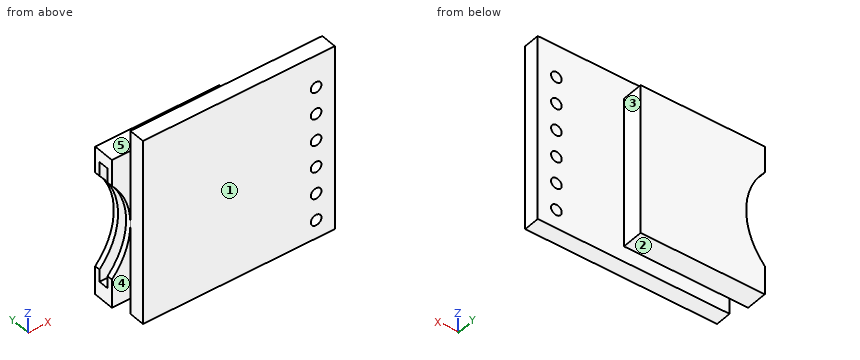
from build123d import *

# Parameters (mm, degrees)
SKETCH1_W           = 18
SKETCH1_H           = 17.5
BOSS_EXTRUDE1_DEPTH = 1.5
BOSS_EXTRUDE2_DEPTH = 2
SKETCH3_R           = 0.5
CUT_EXTRUDE1_DEPTH  = 2.5
SKETCH4_W           = 11.451958773
SKETCH4_H           = 0.968573627
CUT_EXTRUDE2_DEPTH  = 9.649638


with BuildPart() as part:
    # Sketch1 → Boss-Extrude1 (new body)
    with BuildSketch(Plane(origin=(0, 0, 0), x_dir=(1, 0, 0), z_dir=(0, 1, 0))):
        with Locations((9, 8.75)):
            Rectangle(SKETCH1_W, SKETCH1_H)
    extrude(amount=BOSS_EXTRUDE1_DEPTH)

    # Sketch2 → Boss-Extrude2 (add)
    with BuildSketch(Plane(origin=(0, 1.5, 0), x_dir=(1, 0, 0), z_dir=(0, 1, 0))):
        with BuildLine():
            Line((-1.742375604, 4.397064227), (-1.742375604, 1.912224032))
            Line((-1.742375604, 1.912224032), (9.907262148, 1.912224032))
            Line((9.907262148, 1.912224032), (9.907262148, 16.039286602))
            Line((9.907262148, 16.039286602), (-1.742375604, 16.039286602))
            Line((-1.742375604, 16.039286602), (-1.742375604, 13.34923012))
            ThreePointArc((-1.742375604, 13.34923012), (0, 8.873147173), (-1.742375604, 4.397064227))
        make_face()
    extrude(amount=BOSS_EXTRUDE2_DEPTH)

    # Sketch3 → Cut-Extrude1 (cut, through all)
    with BuildSketch(Plane(origin=(0, 1.5, 0), x_dir=(1, 0, 0), z_dir=(0, 1, 0))):
        with Locations((16.25, 15.75)):
            Circle(SKETCH3_R)
        with Locations((16.25, 13.21)):
            Circle(SKETCH3_R)
        with Locations((16.25, 10.67)):
            Circle(SKETCH3_R)
        with Locations((16.25, 8.13)):
            Circle(SKETCH3_R)
        with Locations((16.25, 5.59)):
            Circle(SKETCH3_R)
        with Locations((16.25, 3.05)):
            Circle(SKETCH3_R)
    extrude(amount=-CUT_EXTRUDE1_DEPTH, mode=Mode.SUBTRACT)

    # Sketch4 → Cut-Extrude2 (cut)
    with BuildSketch(Plane.ZY.offset(1.742375604)):
        with Locations((-8.77848746, 2.504917681)):
            Rectangle(SKETCH4_W, SKETCH4_H)
    extrude(amount=-CUT_EXTRUDE2_DEPTH, mode=Mode.SUBTRACT)


solid = part.part
Work out the finished part from the listing and answer in its coordinate system (mm). Face numbers are marked on the shaded views. A direction names the side the tool comes from. Give positions to 0.01 mm unless a question says otherwise; leave off trailing zeros. Write each loop counter-clockwise with the first axis right and the second up, starting at its lowest first coordinate (ties: lowest second). Pieces come first, ordered by that corner, then holes. Notation, with made-up numbers: (49, 34) - (55, 34) arc R14 cw to (55, 47) - close; hole circle Ø2 at (39, 55.25). An arc over 180 degrees is marked (long way). One line per item, written item: value. Start each with the question number.
1. Given pin 1 (0.6 mm diameter, centred on x = 2.5, y = 2.5, fed in from -Z); pin 2 (1.4 mm diameter, centred on x = -0.5, z = -11, fed in from -Y); pin 3 (8 mm diameter, centred on x = 16, z = -10.5, fed in from +Y); pin 4 (1 mm diameter, centred on x = 5, y = 3, fed in from +Z), each flat-ended and moving along its own axis, determine where each tip first touches the part or whether it passes through.
2. Consider probe 1 along Y at (x, z) = (5.5, -7.5); probe 2 along X at (y, z) = (1.1, -3.05); probe 3 along Z at (x, y) = (6.5, 2.3). Determine where each line is inside the solid, lowest interval first.
3. Find section D-D (z = -6.75). Write down the section's boundary in (x, y), then the cut area to 3 significant figures.
4. Find section A-A (x = 16.25). Write down the section's boundary in (y, z), then the cut area to 4 significant figures.
5. For the marked faces 1, 2, 3, 4 and 5, determine the directions among +Z, -Z, +X, -X, +Y, -Y from which every point of the face is accessible in a straight line to the end or side of a thin tool.
6. Find section B-B (z = -15.75). Write down the section's boundary in (x, y), then the cut area to 3 significant figures.
7. Find section C-C (x = 2). Write down the section's boundary in (y, z).
Geometry results:
1. pin 1: z = -16.04
1. pin 2: y = 0
1. pin 3: y = 1.5
1. pin 4: z = -1.91
2. probe 1: 0 to 2.02, 2.99 to 3.5
2. probe 2: 0 to 15.75, 16.75 to 18
2. probe 3: -16.04 to -14.5, -3.05 to -1.91
3. outline: (-0.35, 1.5) - (0, 1.5) - (0, 0) - (18, 0) - (18, 1.5) - (9.91, 1.5) - (9.91, 3.5) - (-0.35, 3.5) - (-0.35, 2.99) - (7.91, 2.99) - (7.91, 2.02) - (-0.35, 2.02) - close
3. area: 39.5 mm2
4. outline: (0, -17.5) - (1.5, -17.5) - (1.5, -16.25) - (0, -16.25) - close; (0, -15.25) - (1.5, -15.25) - (1.5, -13.71) - (0, -13.71) - close; (0, -12.71) - (1.5, -12.71) - (1.5, -11.17) - (0, -11.17) - close; (0, -10.17) - (1.5, -10.17) - (1.5, -8.63) - (0, -8.63) - close; (0, -7.63) - (1.5, -7.63) - (1.5, -6.09) - (0, -6.09) - close; (0, -5.09) - (1.5, -5.09) - (1.5, -3.55) - (0, -3.55) - close; (0, -2.55) - (1.5, -2.55) - (1.5, 0) - (0, 0) - close
4. area: 17.25 mm2
5. face 1: +Z, -Z, +X, -X, -Y
5. face 2: -Z, +X, -X, +Y
5. face 3: +Z, -Z, +X, +Y
5. face 4: +Z, -Z, -X, -Y
5. face 5: +Z, +X, -X, +Y
6. outline: (-1.74, 1.5) - (0, 1.5) - (0, 0) - (15.75, 0) - (15.75, 1.5) - (9.91, 1.5) - (9.91, 3.5) - (-1.74, 3.5) - close; (16.75, 0) - (18, 0) - (18, 1.5) - (16.75, 1.5) - close
6. area: 48.8 mm2
7. outline: (0, -17.5) - (1.5, -17.5) - (1.5, -16.04) - (3.5, -16.04) - (3.5, -1.91) - (1.5, -1.91) - (1.5, 0) - (0, 0) - close; hole (2.02, -14.5) - (2.99, -14.5) - (2.99, -3.05) - (2.02, -3.05) - close
